```python
from build123d import *

# Parameters (mm, degrees)
SKETCH_1_W          = 9.5
SKETCH_1_H          = 9.5
EXTRUDE_1_DEPTH     = 3.3
SKETCH_2_W          = 9.5
SKETCH_2_H          = 6
EXTRUDE_2_DEPTH     = 1.2
SKETCH_3_R          = 2.5
CUT_EXTRUDE_1_DEPTH = 5.5
CUT_EXTRUDE_2_DEPTH = 10.5


with BuildPart() as part:
    # 草图1 → 凸台-拉伸1 (new body)
    with BuildSketch(Plane(origin=(0, 0, 0), x_dir=(1, 0, 0), z_dir=(0, 1, 0))):
        with Locations((4.75, 4.75)):
            Rectangle(SKETCH_1_W, SKETCH_1_H)
    extrude(amount=EXTRUDE_1_DEPTH)

    # 草图2 → 凸台-拉伸2 (add)
    with BuildSketch(Plane(origin=(0, 3.3, 0), x_dir=(1, 0, 0), z_dir=(0, 1, 0))):
        with Locations((4.75, 4.75)):
            Rectangle(SKETCH_2_W, SKETCH_2_H)
    extrude(amount=EXTRUDE_2_DEPTH)

    # 草图3 → 切除-拉伸1 (cut, through all)
    with BuildSketch(Plane(origin=(0, 4.5, 0), x_dir=(1, 0, 0), z_dir=(0, 1, 0))):
        with Locations((4.75, 4.75)):
            Circle(SKETCH_3_R)
    extrude(amount=-CUT_EXTRUDE_1_DEPTH, mode=Mode.SUBTRACT)

    # 草图4 → 切除-拉伸2 (cut, through all)
    with BuildSketch(Plane.ZY):
        Polygon((-9.5, 2.3), (-7.2, 0), (-9.5, 0), align=None)
        Polygon((0, 2.3), (-2.3, 0), (0, 0), align=None)
    extrude(amount=-CUT_EXTRUDE_2_DEPTH, mode=Mode.SUBTRACT)


solid = part.part
```
Could you check a few things on this model? Use its own coordinates, in mm. A direction names the side the tool comes from. Give positions to 0.01 mm unless a question says otherwise; leave off trailing zeros. Order: outer loops, then holes, each group sorted by start corner. A loop starts at its lowest first (then second) coordinate and runs counter-clockwise, first axis right, second up.
Q1. If I drill on line 1 along X through (y, z) = (0.8, -4.75); line 2 along Z through (x, y) = (4.75, 3.45); line 3 along X through (y, z) = (3.05, -5.5), over which ranges is the centre line in solid material (lowest first)?
Q2. We'd pull the mould along Z, two halves only. Please class faces 4 (the cylindrical face through (7.135, 2.282, -5.501)), 5 (the flat face through (0, 2, -5)), 6 (the flat face through (5, 4, -7.75)): +Z half, -Z half, draft (parallel to the pull), parting line (faces both ways), or undercut.
Q3. Suppose I cut it at A-A, the plane x = 4.75. Write out the boundary of the cut face in (y, z).
Q4. For faces 1 (the flat face through (5, 3.3, -9)), 2 (the flat face through (5, 3.3, -1)), 3 (the flat face through (4.7, 1.2, -8.4)), which set-ups out of +Z, -Z, +X, -X, +Y, -Y let a thin tool reach every point of the face, with its end or its side?
Q5. I'm going to push flat-ended pins straight in: P1, Ø2, axis at x = 7.5, z = -5, coming from the -Y side; P2, Ø0.6, axis at x = 6.5, y = 4, coming from the +Z side; P3, Ø0.5, axis at x = 6.5, z = -9, coming from the +Y side; P4, Ø3, axis at x = 4.5, z = -5, coming from the -Y side. Where does each tip first touch, or does it pass through?
Q6. Suppose I cut it at B-B, the plane z = -4.75. Write out the boundary of the cut face in (x, y), and give its area (4 significant figures).
Q7. Suppose I cut it at C-C, the plane y = 4.25. Write out the boundary of the cut face in (x, z), and give its area (3 significant figures).
Q8. Suppose I cut it at D-D, the plane x = 2.5. Write out the boundary of the cut face in (y, z).
Solution:
1. line 1: x = 0 to 2.25, 7.25 to 9.5
1. line 2: z = -7.75 to -7.25, -2.25 to -1.75
1. line 3: x = 0 to 2.37, 7.13 to 9.5
2. face 4: undercut
2. face 5: draft
2. face 6: -Z half
3. outline: (0.05, -7.25) - (2.3, -9.5) - (3.3, -9.5) - (3.3, -7.75) - (4.5, -7.75) - (4.5, -7.25) - close; (0.05, -2.25) - (4.5, -2.25) - (4.5, -1.75) - (3.3, -1.75) - (3.3, 0) - (2.3, 0) - close
4. face 1: -Z, +X, -X, +Y
4. face 2: +Z, +X, -X, +Y
4. face 3: -Z, +X, -X, -Y
5. P1: stops at y = 0
5. P2: stops at z = -1.75
5. P3: stops at y = 3.3
5. P4: passes through
6. outline: (0, 0) - (2.25, 0) - (2.25, 4.5) - (0, 4.5) - close; (7.25, 0) - (9.5, 0) - (9.5, 4.5) - (7.25, 4.5) - close
6. area: 20.25 mm2
7. outline: (0, -7.75) - (9.5, -7.75) - (9.5, -1.75) - (0, -1.75) - close; hole circle Ø5 at (4.75, -4.75)
7. area: 37.4 mm2
8. outline: (0, -7.2) - (2.3, -9.5) - (3.3, -9.5) - (3.3, -7.75) - (4.5, -7.75) - (4.5, -5.84) - (0, -5.84) - close; (0, -3.66) - (4.5, -3.66) - (4.5, -1.75) - (3.3, -1.75) - (3.3, 0) - (2.3, 0) - (0, -2.3) - close
